Verification items for this drawing (mm, ordinates from the low corner). Round coordinates to 2 decimals unless told otherwise and drop trailing zeros. Order: outer loops, then holes, each group sorted by start corner. A loop starts at its lowest first (then second) coordinate and runs counter-clockwise, first axis right, second up. Notation, with made-up numbers: M 64,32.5 L 121,32.5 A16 cw 121,56.5 Z; hole C 14,-8 d8. An arc over 180 degrees is marked long. Use CSV: the item, a comma, the result in double quotes. Start each with the question number.
Q1. Sectioned sample at B-B (x = 35). Enter the section's corners in (y, z), and give its area (3 significant figures).
Q2. Gauge pin test, flat end, axial feed: pin 1 Ø25 at (x, z) = (13, 524) entering from +Y. Record the tip position at first contact, or that the pin passes through.
Q3. Sectioned sample at A-A (y = 47.5). Enter the section's corners in (x, z).
Q4. Mould release check, pull along Z, two halves, no side actions. Record for the marked faces 1, 2 and 3: +Z half, -Z half, draft (parallel to the pull), parting line (faces both ways), or undercut.
Q5. Scan lines: line 1 (Z direction, x = 27.5, y = 57.5); line 2 (Y direction, x = 33, z = 536). Record each from-to range of solid material in increasing order.
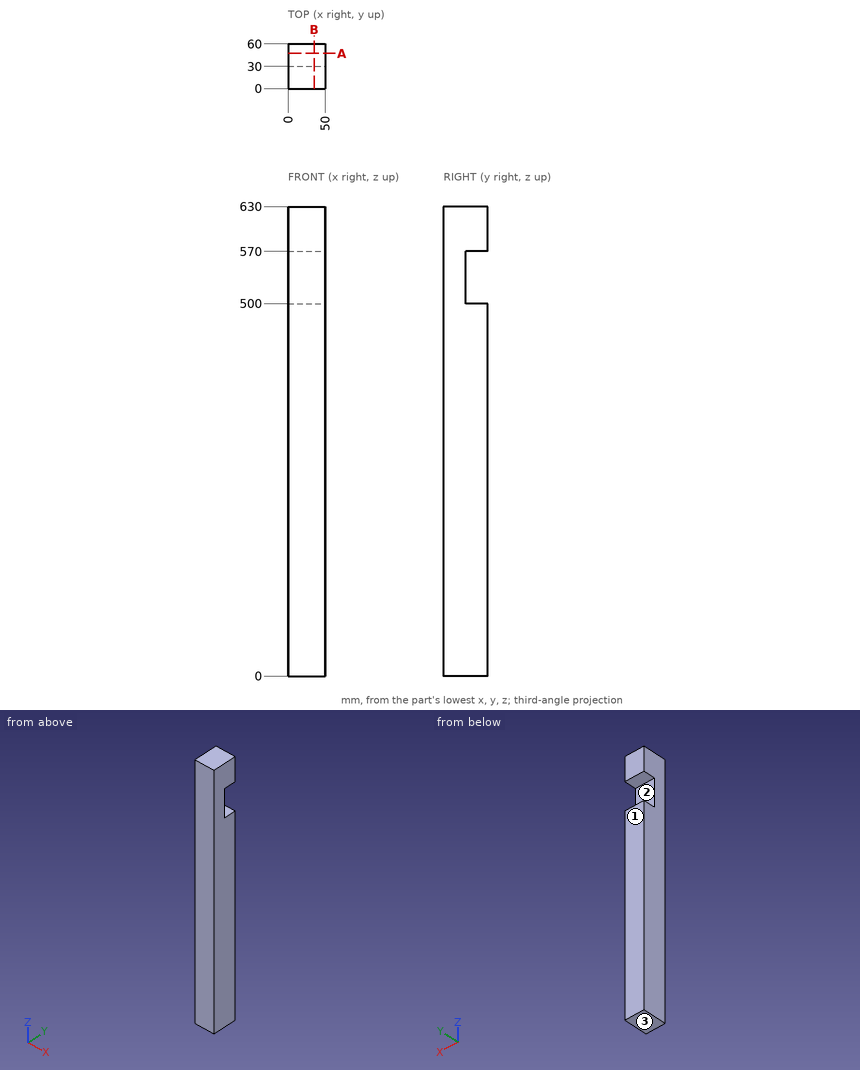
Verdict:
1,outline,"M 0,0 L 60,0 L 60,500 L 30,500 L 30,570 L 60,570 L 60,630 L 0,630 Z"
1,area,"35,700 mm²"
2,pin 1,"stops at y = 30"
3,outline,"M 0,0 L 50,0 L 50,500 L 0,500 Z; M 0,570 L 50,570 L 50,630 L 0,630 Z"
4,face 1,"draft"
4,face 2,"undercut"
4,face 3,"-Z half"
5,line 1,"z = 0 to 500, 570 to 630"
5,line 2,"y = 0 to 30"
